Read the model definition and answer for the solid it produces. Units are mm, in the model's axes. A direction names the side the tool comes from. Coordinates: 2 decimals unless noted, no trailing zeros. Write each loop counter-clockwise with the first axis right and the second up, starting at its lowest first coordinate (ties: lowest second). Pieces come first, ordered by that corner, then holes. Notation, with made-up numbers: (52.5, 66.5) -> (76.5, 66.5) arc R30 ccw to (76.5, 94.5) -> close; hole circle Ø2 at (7.25, 7.5). An arc over 180 degrees is marked (long way). Answer in a Markdown table with one row per item. Add a question column.
Item 1: Section B-B on y = 0 is taken. Write down the section's boundary in (x, z).
Item 2: Given pin 1 Ø4 at (y, z) = (-1, 1.5) entering from -X; pin 2 Ø5 at (x, z) = (-3, 5.5) entering from -Y; pin 3 Ø13 at (y, z) = (0, 0) entering from -X; pin 4 Ø1.5 at (y, z) = (29.5, 5) entering from -X, each flat-ended and moving along its own axis, determine where each tip first touches the part or whether it passes through.
Item 3: Straight lines are drawn through the part: line 1 (Y direction, x = 0, z = -4); line 2 (Y direction, x = -3, z = 3.5); line 3 (Y direction, x = -21.5, z = 1.5). For each, find the intervals that lie inside material, in ascending order. Write a range as from..to.
Item 4: Section D-D on x = -39.5 is taken. Write down the section's boundary in (y, z), then the cut area to 3 significant figures.
Item 5: Which of the six approach directions +Z, -Z, +X, -X, +Y, -Y give full straight-line access (tool end or side, diameter ignored) to faces 4 (the face through (52.535, -3.905, 0.867)), 5 (the face through (-14.985, 0.66, -8.958)), 6 (the face through (43.389, -24.847, 0.084))?
Item 6: For a pull along Z with two mould halves and no side action, classify faces 1 (the face through (-23.347, -47.183, -2.15)), 2 (the face through (16.414, -45.11, 0.084)), 3 (the face through (3, -10, 12)) as +Z half, -Z half, draft (parallel to the pull), parting line (faces both ways), or undercut.
Item 7: Section C-C on y = -29 is taken. Write down the section's boundary in (x, z), then the cut area to 3 significant figures.
Item 8: Section A-A on x = 0 is taken. Write down the section's boundary in (y, z).
```python
from build123d import *

# Parameters (mm, degrees)
CROQUIS1_R              = 15
CROQUIS1_R_2            = 10
SALIENTE_EXTRUIR1_DEPTH = 12
CROQUIS2_R              = 55
CROQUIS2_R_2            = 15
SALIENTE_EXTRUIR2_DEPTH = 6
CROQUIS4_R              = 4
CORTAR_EXTRUIR2_DEPTH   = 5
MATRIZC1_COUNT          = 6


with BuildPart() as part:
    # Croquis1 → Saliente-Extruir1 (new, symmetric)
    with BuildSketch(Plane.XY):
        Circle(CROQUIS1_R)
        Circle(CROQUIS1_R_2, mode=Mode.SUBTRACT)
    extrude(amount=SALIENTE_EXTRUIR1_DEPTH, both=True)

    # Croquis2 → Saliente-Extruir2 (add, symmetric)
    with BuildSketch(Plane.XY):
        Circle(CROQUIS2_R)
        Circle(CROQUIS2_R_2, mode=Mode.SUBTRACT)
        with BuildLine():
            Line((-16.39599659, 40.077890975), (-7.597218099, 21.20884961))
            ThreePointArc((-7.597218099, 21.20884961), (-6.21113479, 19.789040466), (-4.241995424, 19.544960343))
            ThreePointArc((-4.241995424, 19.544960343), (0, 20), (4.241995424, 19.544960343))
            ThreePointArc((4.241995424, 19.544960343), (6.21113479, 19.789040466), (7.597218099, 21.20884961))
            Line((7.597218099, 21.20884961), (16.39599659, 40.077890975))
            ThreePointArc((16.39599659, 40.077890975), (16.383120253, 45.176742429), (12.452443031, 48.424546075))
            ThreePointArc((12.452443031, 48.424546075), (0, 50), (-12.452443031, 48.424546075))
            ThreePointArc((-12.452443031, 48.424546075), (-16.383120253, 45.176742429), (-16.39599659, 40.077890975))
        make_face(mode=Mode.SUBTRACT)
        with BuildLine():
            Line((42.90647001, 5.83959592), (22.166011596, 4.025040933))
            ThreePointArc((22.166011596, 4.025040933), (20.243379154, 4.515519719), (19.047429885, 6.098804372))
            ThreePointArc((19.047429885, 6.098804372), (17.320508076, 10), (14.805434461, 13.446155972))
            ThreePointArc((14.805434461, 13.446155972), (14.032244365, 15.273520747), (14.568793497, 17.183808677))
            Line((14.568793497, 17.183808677), (26.51047342, 34.238295055))
            ThreePointArc((26.51047342, 34.238295055), (30.932646477, 36.776569547), (35.710665552, 34.996405042))
            ThreePointArc((35.710665552, 34.996405042), (43.301270189, 25), (48.163108583, 13.428141033))
            ThreePointArc((48.163108583, 13.428141033), (47.31576673, 8.400172882), (42.90647001, 5.83959592))
        make_face(mode=Mode.SUBTRACT)
        with BuildLine():
            Line((26.51047342, -34.238295055), (14.568793497, -17.183808677))
            ThreePointArc((14.568793497, -17.183808677), (14.032244365, -15.273520747), (14.805434461, -13.446155972))
            ThreePointArc((14.805434461, -13.446155972), (17.320508076, -10), (19.047429885, -6.098804372))
            ThreePointArc((19.047429885, -6.098804372), (20.243379154, -4.515519719), (22.166011596, -4.025040933))
            Line((22.166011596, -4.025040933), (42.90647001, -5.83959592))
            ThreePointArc((42.90647001, -5.83959592), (47.31576673, -8.400172882), (48.163108583, -13.428141033))
            ThreePointArc((48.163108583, -13.428141033), (43.301270189, -25), (35.710665552, -34.996405042))
            ThreePointArc((35.710665552, -34.996405042), (30.932646477, -36.776569547), (26.51047342, -34.238295055))
        make_face(mode=Mode.SUBTRACT)
        with BuildLine():
            Line((-16.39599659, -40.077890975), (-7.597218099, -21.20884961))
            ThreePointArc((-7.597218099, -21.20884961), (-6.21113479, -19.789040466), (-4.241995424, -19.544960343))
            ThreePointArc((-4.241995424, -19.544960343), (0, -20), (4.241995424, -19.544960343))
            ThreePointArc((4.241995424, -19.544960343), (6.21113479, -19.789040466), (7.597218099, -21.20884961))
            Line((7.597218099, -21.20884961), (16.39599659, -40.077890975))
            ThreePointArc((16.39599659, -40.077890975), (16.383120253, -45.176742429), (12.452443031, -48.424546075))
            ThreePointArc((12.452443031, -48.424546075), (0, -50), (-12.452443031, -48.424546075))
            ThreePointArc((-12.452443031, -48.424546075), (-16.383120253, -45.176742429), (-16.39599659, -40.077890975))
        make_face(mode=Mode.SUBTRACT)
        with BuildLine():
            Line((-42.90647001, -5.83959592), (-22.166011596, -4.025040933))
            ThreePointArc((-22.166011596, -4.025040933), (-20.243379154, -4.515519719), (-19.047429885, -6.098804372))
            ThreePointArc((-19.047429885, -6.098804372), (-17.320508076, -10), (-14.805434461, -13.446155972))
            ThreePointArc((-14.805434461, -13.446155972), (-14.032244365, -15.273520747), (-14.568793497, -17.183808677))
            Line((-14.568793497, -17.183808677), (-26.51047342, -34.238295055))
            ThreePointArc((-26.51047342, -34.238295055), (-30.932646477, -36.776569547), (-35.710665552, -34.996405042))
            ThreePointArc((-35.710665552, -34.996405042), (-43.301270189, -25), (-48.163108583, -13.428141033))
            ThreePointArc((-48.163108583, -13.428141033), (-47.31576673, -8.400172882), (-42.90647001, -5.83959592))
        make_face(mode=Mode.SUBTRACT)
        with BuildLine():
            Line((-26.51047342, 34.238295055), (-14.568793497, 17.183808677))
            ThreePointArc((-14.568793497, 17.183808677), (-14.032244365, 15.273520747), (-14.805434461, 13.446155972))
            ThreePointArc((-14.805434461, 13.446155972), (-17.320508076, 10), (-19.047429885, 6.098804372))
            ThreePointArc((-19.047429885, 6.098804372), (-20.243379154, 4.515519719), (-22.166011596, 4.025040933))
            Line((-22.166011596, 4.025040933), (-42.90647001, 5.83959592))
            ThreePointArc((-42.90647001, 5.83959592), (-47.31576673, 8.400172882), (-48.163108583, 13.428141033))
            ThreePointArc((-48.163108583, 13.428141033), (-43.301270189, 25), (-35.710665552, 34.996405042))
            ThreePointArc((-35.710665552, 34.996405042), (-30.932646477, 36.776569547), (-26.51047342, 34.238295055))
        make_face(mode=Mode.SUBTRACT)
    extrude(amount=SALIENTE_EXTRUIR2_DEPTH, both=True)

    # Croquis4 → Cortar-Extruir2 (cut)
    with BuildSketch(Plane(origin=(55, 0, 0), x_dir=(0, 0, -1), z_dir=(1, 0, 0))):
        Circle(CROQUIS4_R)
    cortar_extruir2 = extrude(amount=-CORTAR_EXTRUIR2_DEPTH, mode=Mode.SUBTRACT)

    # MatrizC1: Cortar-Extruir2 ×6 about axis
    matrizc1_axis = Axis((0, 0, 0), (0, 0, 1))
    for i in range(1, MATRIZC1_COUNT):
        add(cortar_extruir2.rotate(matrizc1_axis, i * 360 / MATRIZC1_COUNT), mode=Mode.SUBTRACT)


solid = part.part
```
Results below:
| question | item | result |
|---|---|---|
| 1 | outline | (-55, -6) -> (-15, -6) -> (-15, -12) -> (-10, -12) -> (-10, 12) -> (-15, 12) -> (-15, 6) -> (-55, 6) -> (-55, 4) -> (-50, 4) -> (-50, -4) -> (-55, -4) -> close; (10, -12) -> (15, -12) -> (15, -6) -> (55, -6) -> (55, -4) -> (50, -4) -> (50, 4) -> (55, 4) -> (55, 6) -> (15, 6) -> (15, 12) -> (10, 12) -> close |
| 2 | pin 1 | stops at x = -50 |
| 2 | pin 2 | stops at y = -55 |
| 2 | pin 3 | stops at x = -55 |
| 2 | pin 4 | stops at x = -46.89 |
| 3 | line 1 | y = -55..-50, -20..-10, 10..20, 50..55 |
| 3 | line 2 | y = -54.92..-49.91, -19.77..-9.54, 9.54..19.77, 49.91..54.92 |
| 3 | line 3 | y = -50.62..-27.08, -4.04..4.04, 27.08..50.62 |
| 4 | outline | (-38.27, -6) -> (-30.66, -6) -> (-30.66, 6) -> (-38.27, 6) -> close; (-5.54, -6) -> (5.54, -6) -> (5.54, 6) -> (-5.54, 6) -> close; (30.66, -6) -> (38.27, -6) -> (38.27, 6) -> (30.66, 6) -> close |
| 4 | area | 316 mm2 |
| 5 | face 4 | +X |
| 5 | face 5 | -Z |
| 5 | face 6 | +Z, -Z |
| 6 | face 1 | undercut |
| 6 | face 2 | draft |
| 6 | face 3 | +Z half |
| 7 | outline | (-46.73, -6) -> (-40.73, -6) -> (-40.73, 6) -> (-46.73, 6) -> close; (-22.84, -6) -> (-11.23, -6) -> (-11.23, 6) -> (-22.84, 6) -> close; (11.23, -6) -> (22.84, -6) -> (22.84, 6) -> (11.23, 6) -> close; (40.73, -6) -> (46.73, -6) -> (46.73, 6) -> (40.73, 6) -> close |
| 7 | area | 423 mm2 |
| 8 | outline | (-55, -6) -> (-50, -6) -> (-50, 6) -> (-55, 6) -> close; (-20, -6) -> (-15, -6) -> (-15, -12) -> (-10, -12) -> (-10, 12) -> (-15, 12) -> (-15, 6) -> (-20, 6) -> close; (10, -12) -> (15, -12) -> (15, -6) -> (20, -6) -> (20, 6) -> (15, 6) -> (15, 12) -> (10, 12) -> close; (50, -6) -> (55, -6) -> (55, 6) -> (50, 6) -> close |
